Build history of the part. All positions in model axes, mm. Face numbers are marked on the shaded views. A direction names the side the tool comes from. Give positions to 0.01 mm unless a question says otherwise; leave off trailing zeros. Order: outer loops, then holes, each group sorted by start corner. A loop starts at its lowest first (then second) coordinate and runs counter-clockwise, first axis right, second up. Notation, with made-up numbers: (-38.75, -3.5) - (11.25, -3.5) arc R36 ccw to (11.25, 31.5) - close; hole circle Ø7 at (18.5, 47). An arc over 180 degrees is marked (long way). Answer in a Markdown table with one row per item.
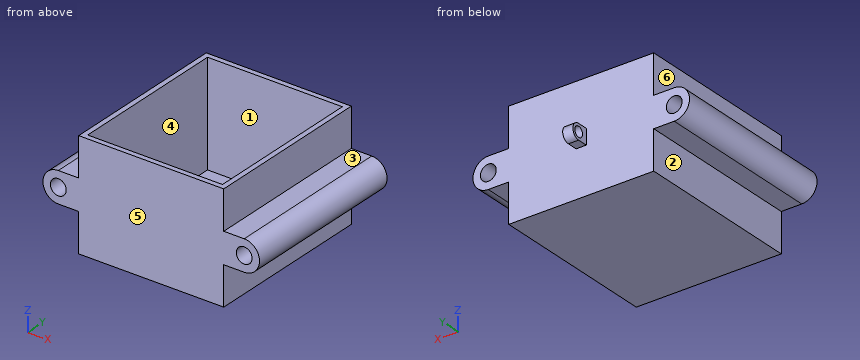
```python
from build123d import *

# Parameters (mm, degrees)
SKETCH_2_W      = 142
SKETCH_2_H      = 166
EXTRUDE_1_DEPTH = 106
SHELL_1_T       = -5
SKETCH_3_R      = 15
SKETCH_3_R_2    = 7.75
EXTRUDE_2_DEPTH = 166
SKETCH_4_R      = 5
EXTRUDE_3_DEPTH = 5


with BuildPart() as part:
    # 스케치2 → 보스-돌출1 (new body)
    with BuildSketch(Plane.XY):
        with Locations((71, 83)):
            Rectangle(SKETCH_2_W, SKETCH_2_H)
    extrude(amount=EXTRUDE_1_DEPTH)

    # 쉘1
    shell_1_openings = [part.faces().sort_by_distance(p)[0] for p in [
        (71, 83, 106),
    ]]
    offset(amount=SHELL_1_T, openings=shell_1_openings, kind=Kind.INTERSECTION)

    # 스케치3 → 보스-돌출2 (add)
    # profile 1 of 4: a face of its own
    with BuildSketch(Plane(origin=(0, 166, 0), x_dir=(1, 0, 0), z_dir=(0, 1, 0))):
        with Locations((-20, -53)):
            Circle(SKETCH_3_R)
        with Locations(Location((-20, -53, 0), (0, 0, 270))):
            Circle(SKETCH_3_R_2, mode=Mode.SUBTRACT)
    # profile 2 of 4: a face of its own
    with BuildSketch(Plane(origin=(0, 166, 0), x_dir=(1, 0, 0), z_dir=(0, 1, 0))):
        with BuildLine():
            Line((0, -38), (-20, -38))
            ThreePointArc((-20, -38), (-9.393398282, -42.393398282), (-5, -53))
            ThreePointArc((-5, -53), (-9.393398282, -63.606601718), (-20, -68))
            Line((-20, -68), (0, -68))
            Line((0, -68), (0, -38))
        make_face()
    # profile 3 of 4: a face of its own
    with BuildSketch(Plane(origin=(0, 166, 0), x_dir=(1, 0, 0), z_dir=(0, 1, 0))):
        with BuildLine():
            ThreePointArc((162, -68), (147, -53), (162, -38))
            Line((162, -38), (142, -38))
            Line((142, -38), (142, -68))
            Line((142, -68), (162, -68))
        make_face()
    # profile 4 of 4: a face of its own
    with BuildSketch(Plane(origin=(0, 166, 0), x_dir=(1, 0, 0), z_dir=(0, 1, 0))):
        with Locations((162, -53)):
            Circle(SKETCH_3_R)
        with Locations(Location((162, -53, 0), (0, 0, 270))):
            Circle(SKETCH_3_R_2, mode=Mode.SUBTRACT)
    extrude(amount=-EXTRUDE_2_DEPTH)

    # 스케치4 → 보스-돌출3 (add, symmetric)
    with BuildSketch(Plane(origin=(71, 0, 0), x_dir=(0, 0, -1), z_dir=(1, 0, 0))):
        with BuildLine():
            ThreePointArc((-45.5, 176), (-53, 183.5), (-60.5, 176))
            Line((-60.5, 176), (-60.5, 166))
            Line((-60.5, 166), (-45.5, 166))
            Line((-45.5, 166), (-45.5, 176))
        make_face()
        with Locations((-53, 176)):
            Circle(SKETCH_4_R, mode=Mode.SUBTRACT)
    extrude(amount=EXTRUDE_3_DEPTH, both=True)


solid = part.part
```
1. Which spindle directions (+Z, -Z, +X, -X, +Y, -Y) get a long thin tool onto all of the face, cutting with end or side? Do the marked faces 1, 2 and 3. Say none if no direction does.
Check result:
| item | result |
|---|---|
| face 1 | +Z |
| face 2 | -Z, -X, +Y, -Y |
| face 3 | +Z, +X, +Y, -Y |
2. Cut at D-D on x = 133.5. Write the cut outline in (y, z).
Check result:
| item | result |
|---|---|
| outline | (0, 0) - (166, 0) - (166, 106) - (161, 106) - (161, 5) - (5, 5) - (5, 106) - (0, 106) - close |
3. Cut at B-B on y = 61. Write the cut outline in (x, z), and give its area (3 significant figures).
Check result:
| item | result |
|---|---|
| outline | (-20, 38) - (0, 38) - (0, 0) - (142, 0) - (142, 38) - (162, 38) arc R15 ccw to (162, 68) - (142, 68) - (142, 106) - (137, 106) - (137, 5) - (5, 5) - (5, 106) - (0, 106) - (0, 68) - (-20, 68) arc R15 ccw to start; hole circle Ø15.5 at (-20, 53); hole circle Ø15.5 at (162, 53) |
| area | 3,250 mm² |
4. Cut at C-C on z = 12. Write the cut outline in (x, y), and give its area (3 significant figures).
Check result:
| item | result |
|---|---|
| outline | (0, 0) - (142, 0) - (142, 166) - (0, 166) - close; hole (5, 5) - (137, 5) - (137, 161) - (5, 161) - close |
| area | 2,980 mm² |
5. Two-plate mould, pull along Y, no slides. Class the marked faces 4, 5 and 6: +Y half, -Y half, draft (parallel to the pull), parting line (faces both ways), or undercut.
Check result:
| item | result |
|---|---|
| face 4 | undercut |
| face 5 | -Y half |
| face 6 | draft |
6. Drop flat-ended pins along their axis: P1, Ø7.5, axis at y = 171, z = 52, coming from the -X side; P2, Ø9.5, axis at x = 162, z = 53, coming from the -Y side; P3, Ø22, axis at x = -9.5, y = 53, coming from the -Z side; P4, Ø3, axis at x = 71, y = 171.5, coming from the +Z side. Give the stop position or say it passes through.
Check result:
| item | result |
|---|---|
| P1 | stops at x = 66 |
| P2 | passes through |
| P3 | stops at z = 0 |
| P4 | stops at z = 60.5 |
7. Cut at A-A on z = 53. Write the cut outline in (x, y).
Check result:
| item | result |
|---|---|
| outline | (-35, 0) - (-27.75, 0) - (-27.75, 166) - (-35, 166) - close; (-12.25, 0) - (154.25, 0) - (154.25, 166) - (76, 166) - (76, 171) - (66, 171) - (66, 166) - (-12.25, 166) - close; (66, 181) - (76, 181) - (76, 183.5) - (66, 183.5) - close; (169.75, 0) - (177, 0) - (177, 166) - (169.75, 166) - close; hole (5, 5) - (137, 5) - (137, 161) - (5, 161) - close |
8. Probe line 1 (X direction, y = 53, z = 53); line 2 (Y direction, x = 73, z = 53); line 3 (X direction, y = 17.5, z = 76). List the from-to ranges inside material, lowest first.
Check result:
| item | result |
|---|---|
| line 1 | x = -35 to -27.75, -12.25 to 5, 137 to 154.25, 169.75 to 177 |
| line 2 | y = 0 to 5, 161 to 171, 181 to 183.5 |
| line 3 | x = 0 to 5, 137 to 142 |
